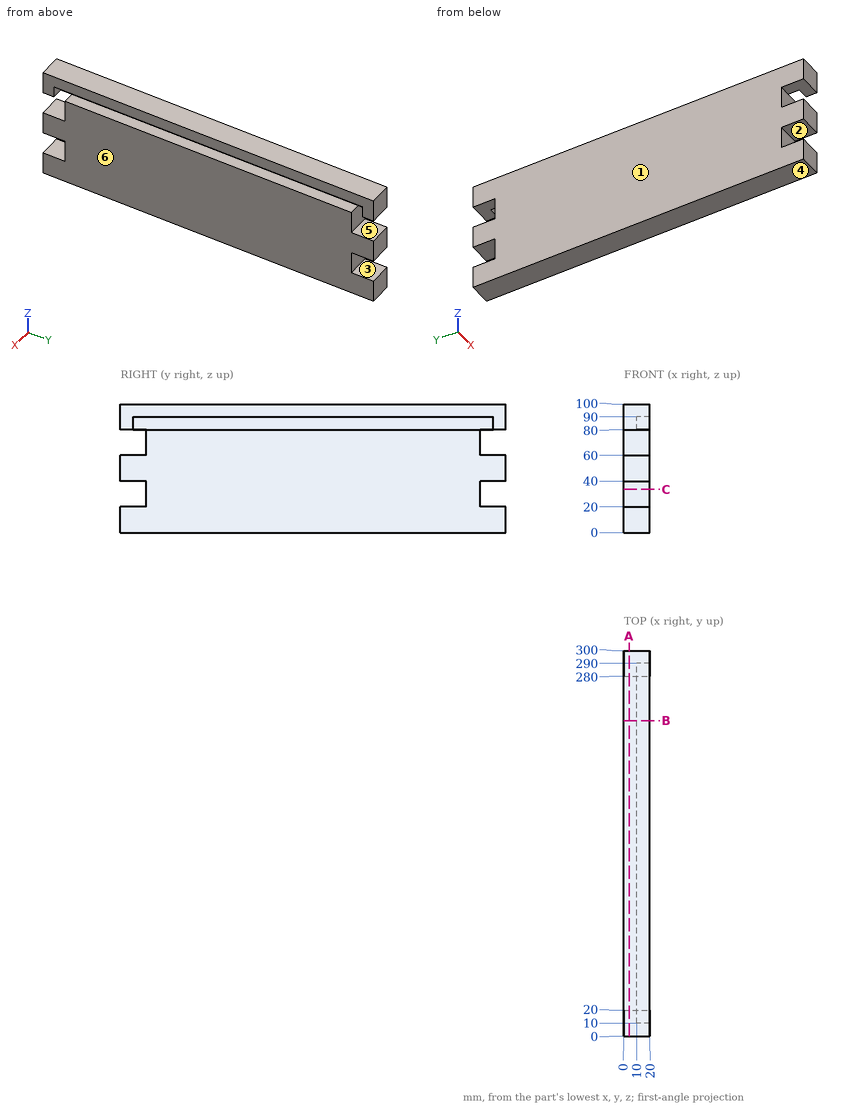
The figure shows three views and two pictorial views of one solid part (mm, origin at its lowest corner). Answer the questions. A direction names the side the tool comes from. Coordinates: 2 decimals unless noted, no trailing zeros. Loops run counter-clockwise (first coordinate to the right, second up) from the corner with the lowest first, then second, coordinate; pieces in that order, holes last. Notation, with made-up numbers: (32, 50.5) -> (60, 50.5) arc R23 cw to (60, 72.5) -> close; hole circle Ø8 at (81.5, 41.5). An arc over 180 degrees is marked (long way). Use one line per item in the form item = value. Start each with the question number.
Item 1: A flat-ended cylindrical pin translates along its axis: pin 1 Ø10 at (x, z) = (13, 30.5) entering from +Y. Find the tip coordinate at first contact, or state that the pin passes through.
Item 2: A tool of negligible diameter and unlimited length cuts with its end or side. For the marked faces 1 and 2, from which of +Z, -Z, +X, -X, +Y, -Y can it reach the whole face along a straight path? Write none if from no direction.
Item 3: The mould has two halves that part along Z. Classify the marked faces 3, 4, 5 and 6: released by +Z, released by -Z, zero draft, split by the parting line, or undercut.
Item 4: Consider L1, parallel to Z at x = 8.25, y = 19; L2, parallel to Z at x = 11, y = 162; L3, parallel to Z at x = 19, y = 14. Determine where each line is inside the solid, lowest interval first. Write a range as [from, to].
Item 5: The part is cut by section B-B on y = 245.5. Determine the outline of the cut face in (x, z), then the cut area to 3 significant figures.
Item 6: The part is cut by section C-C on z = 33.5. Determine the outline of the cut face in (x, y).
Item 7: The part is cut by section A-A on x = 4. Determine the outline of the cut face in (y, z), then the cut area to 3 significant figures.
Answer key:
q1.pin_1 = 280
q2.face_1 = +Z, -Z, -X, +Y, -Y
q2.face_2 = +X, -X, -Y
q3.face_3 = undercut
q3.face_4 = released by -Z
q3.face_5 = undercut
q3.face_6 = zero draft
q4.L1 = [0, 20], [40, 60], [80, 100]
q4.L2 = [0, 80], [90, 100]
q4.L3 = [0, 20], [40, 60], [90, 100]
q5.outline = (0, 0) -> (20, 0) -> (20, 80) -> (10, 80) -> (10, 90) -> (20, 90) -> (20, 100) -> (0, 100) -> close
q5.area = 1,900 mm2
q6.outline = (0, 20) -> (20, 20) -> (20, 280) -> (0, 280) -> close
q7.outline = (0, 0) -> (300, 0) -> (300, 20) -> (280, 20) -> (280, 40) -> (300, 40) -> (300, 60) -> (280, 60) -> (280, 80) -> (300, 80) -> (300, 100) -> (0, 100) -> (0, 80) -> (20, 80) -> (20, 60) -> (0, 60) -> (0, 40) -> (20, 40) -> (20, 20) -> (0, 20) -> close
q7.area = 28,400 mm2
